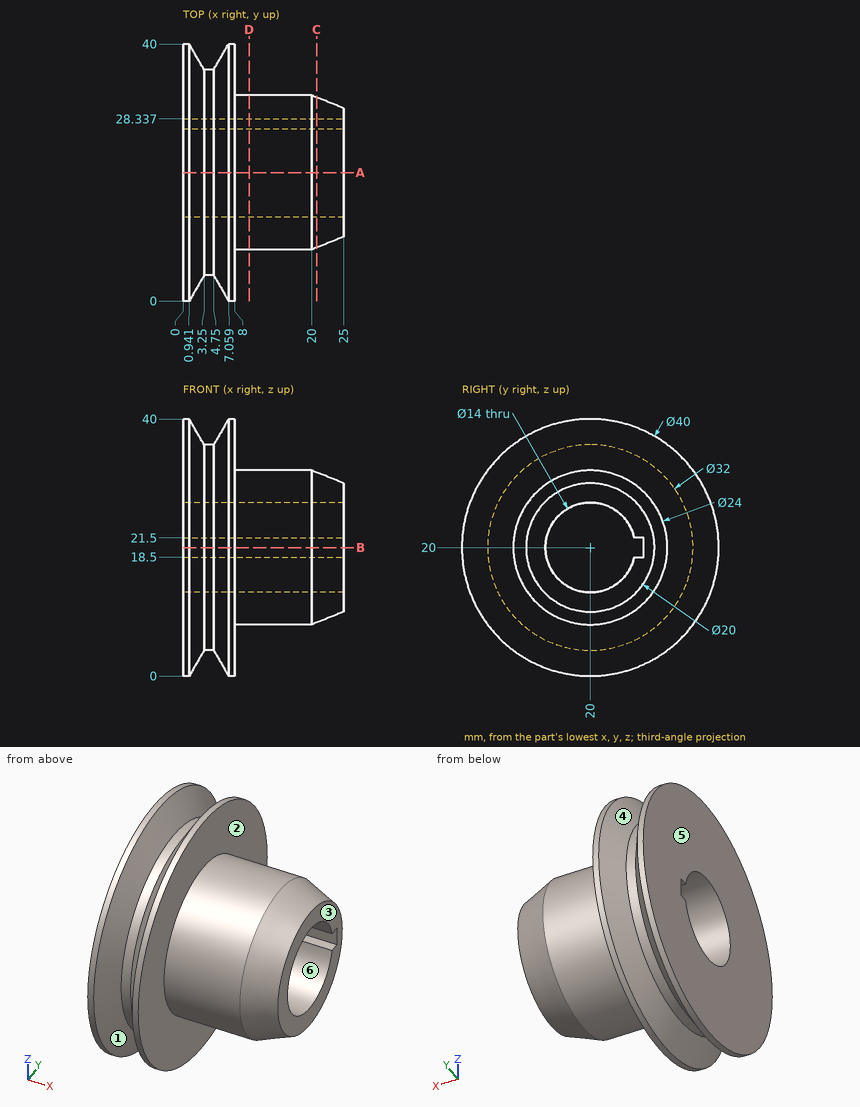
The figure shows three views and two pictorial views of one solid part (mm, origin at its lowest corner). Answer the questions. A direction names the side the tool comes from. Round coordinates to 2 decimals unless told otherwise and drop trailing zeros. Loops run counter-clockwise (first coordinate to the right, second up) from the corner with the lowest first, then second, coordinate; pieces in that order, holes last. Notation, with made-up numbers: M -21,14 L 23,14 A26 ccw 23,44 Z; hole C 82,76 d1. An arc over 180 degrees is marked long. Use CSV: the item, a comma, the result in double quotes.
Q1. Section D-D, the plane x = 10.25 is taken. Determine the outline of the cut face in (y, z), then the cut area to 3 significant figures.
Determined:
outline,"C 20,20 d24; hole M 26.84,18.5 L 28.34,18.5 L 28.34,21.5 L 26.84,21.5 A7 ccw long Z"
area,"294 mm2"
Q2. Consider L1, parallel to Z at x = 14.25, y = 20; L2, parallel to Y at x = 17.75, z = 20; L3, parallel to X at y = 26.5, z = 32.5. Determine where each line is inside the solid, lowest interval first.
Determined:
L1,"8 to 13, 27 to 32"
L2,"8 to 13, 28.34 to 32"
L3,"0 to 8"
Q3. A tool of negligible diameter and unlimited length cuts with its end or side. For the marked faces 1, 2 and 3, from which of +Z, -Z, +X, -X, +Y, -Y can it reach the whole face along a straight path? Write none if from no direction.
Determined:
face 1,"none"
face 2,"+X"
face 3,"+Z, -Z, +X, +Y, -Y"
Q4. The mould has two halves that part along Z. Classify the marked faces 4, 5 and 6: pulls with the +Z half, pulls with the -Z half, needs draft (parallel to the pull), parting line crosses it, or undercut.
Determined:
face 4,"parting line crosses it"
face 5,"needs draft"
face 6,"undercut"
Q5. Section B-B, the plane z = 20 is taken. Determine the outline of the cut face in (x, y), then the cut area to 3 significant figures.
Determined:
outline,"M 0,0 L 0.94,0 L 3.25,4 L 4.75,4 L 7.06,0 L 8,0 L 8,8 L 20,8 L 25,10 L 25,13 L 0,13 Z; M 0,28.34 L 25,28.34 L 25,30 L 20,32 L 8,32 L 8,40 L 7.06,40 L 4.75,36 L 3.25,36 L 0.94,40 L 0,40 Z"
area,"304 mm2"
Q6. Section A-A, the plane y = 20 is taken. Determine the outline of the cut face in (x, z).
Determined:
outline,"M 0,0 L 0.94,0 L 3.25,4 L 4.75,4 L 7.06,0 L 8,0 L 8,8 L 20,8 L 25,10 L 25,13 L 0,13 Z; M 0,27 L 25,27 L 25,30 L 20,32 L 8,32 L 8,40 L 7.06,40 L 4.75,36 L 3.25,36 L 0.94,40 L 0,40 Z"
Q7. Each of these flat-tipped pins is pushed along its axis until it touches: pin 1 (0.8 mm diameter, centred on x = 16.5, y = 27.5, fed in from +Z) (1 decimal); pin 2 (1.7 mm diameter, centred on x = 18, y = 27.5, fed in from -Z); pin 3 (3.5 mm diameter, centred on x = 8.5, z = 20, fed in from -Y). Where does it stop, or does it pass through?
Determined:
pin 1,"z = 29.7"
pin 2,"z = 10.01"
pin 3,"y = 0"
Q8. Section C-C, the plane x = 20.75 is taken. Determine the outline of the cut face in (y, z), then the cut area to 3 significant figures.
Determined:
outline,"C 20,20 d23.4; hole M 26.84,18.5 L 28.34,18.5 L 28.34,21.5 L 26.84,21.5 A7 ccw long Z"
area,"272 mm2"
